from build123d import *

# Parameters (mm, degrees)
F1_DEPTH = 33
F2_R     = 1.1
F2_R_2   = 2
F3_DEPTH = 32.301
F4_R     = 1
F5_R     = 5


with BuildPart() as f1:
    # F0 (on Front) → F1 (new body)
    with BuildSketch(Plane.XZ):
        Polygon((0, 24.5), (0, 0), (1.5, 0), (1.5, 23), (30.8, 23), (30.8, 0), (32.3, 0), (32.3, 24.5), align=None)
    extrude(amount=F1_DEPTH)

    # F2 (on face) → F3 (cut, through all)
    with BuildSketch(Plane(origin=(0, 0, 0), x_dir=(0, -1, 0), z_dir=(-1, 0, 0))):
        with BuildLine():
            Line((0, 8), (0, 0))
            Line((0, 0), (24.5, 0))
            Line((24.5, 0), (24.5, 8))
            Line((24.5, 8), (12.5, 8))
            Line((12.5, 8), (12.5, 10))
            ThreePointArc((12.5, 10), (8.5, 14), (4.5, 10))
            Line((4.5, 10), (4.5, 8))
            Line((4.5, 8), (0, 8))
        make_face()
        with Locations((14.7225396744, 10)):
            Circle(F2_R)
        with Locations((12.9, 14.4)):
            Circle(F2_R)
        with Locations((8.5, 16.2225396744)):
            Circle(F2_R)
        with Locations((4.1, 14.4)):
            Circle(F2_R)
        with Locations((2.2774603256, 10)):
            Circle(F2_R)
        with Locations((28.5, 3)):
            Circle(F2_R_2)
    extrude(amount=-F3_DEPTH, mode=Mode.SUBTRACT)

    # F4
    f4_edges = [f1.edges().sort_by_distance(p)[0] for p in [
        (0.75, -4.5, 8),
        (31.55, -4.5, 8),
        (0.75, -12.5, 8),
        (31.55, -12.5, 8),
        (31.55, 0, 8),
        (0.75, 0, 8),
        (0.75, -24.5, 0),
        (31.55, -24.5, 0),
        (0.75, -33, 0),
        (31.55, -33, 0),
    ]]
    fillet(f4_edges, radius=F4_R)

    # F5
    f5_edges = [f1.edges().sort_by_distance(p)[0] for p in [
        (0.75, -24.5, 8),
        (31.55, -24.5, 8),
    ]]
    fillet(f5_edges, radius=F5_R)


solid = f1.part
The model under review builds one solid part; all positions refer to its coordinate system, in mm. A direction names the side the tool comes from. Round coordinates to 2 decimals unless told otherwise and drop trailing zeros. Order: outer loops, then holes, each group sorted by start corner. A loop starts at its lowest first (then second) coordinate and runs counter-clockwise, first axis right, second up. Notation, with made-up numbers: (35, -4) -> (60, -4) arc R18 ccw to (60, 19) -> close; hole circle Ø6 at (10, 19.25). An arc over 180 degrees is marked (long way). Write item = value, one per line. Start each with the question number.
Item 1: Clearance check with flat-ended pins moving along their axes: pin 1 Ø5 at (x, y) = (15, -16.5) entering from -Z; pin 2 Ø0.8 at (x, y) = (1, -17) entering from -Z; pin 3 Ø1.6 at (x, z) = (31.5, 2) entering from +Y; pin 4 Ø12 at (y, z) = (-11, 4) entering from +X. State where each tip first meets the part, or that it passes through.
Item 2: Consider section D-D on y = -29. Write out the cut boundary in (x, z), plus the area to 3 significant figures.
Item 3: For faces 1 (the face through (32, -17, 8)), 2 (the face through (0.76, -12.785, 8.301)), 3 (the face through (31.54, -4.69, 15.33)), list the 3-axis set-ups (+Z, -Z, +X, -X, +Y, -Y) from which the entire face can be reached by the end or side of a thin tool; tool diameter is ignored.
Item 4: Consider section B-B on z = 18.25. Write out the cut boundary in (x, y), plus the area to 3 significant figures.
Item 5: Consider section C-C on z = 2.5. Write out the cut boundary in (x, y).
Item 6: Consider section A-A on y = -8.5. Write out the cut boundary in (x, z).
Item 7: For line 1 along Z through (x, y) = (1.1, -28.5); line 2 along Z through (x, y) = (3.5, -14); line 3 along X through (y, z) = (-18, 8.5), list the stretches that pass through material, from the lowest coordinate up.
Item 8: Mouldability with a two-part tool opening along Z and no side actions: class faces 4 (the face through (31.56, -12.801, 8.285)), 5 (the face through (31.54, -8.357, 17.313)), 6 (the face through (1, -24.5, 2)) as released by +Z, released by -Z, zero draft, split by the parting line, or undercut.
Conclusion:
q1.pin_1 = 23
q1.pin_2 = 8
q1.pin_3 = -24.5
q1.pin_4 = 32.3
q2.outline = (0, 0) -> (1.5, 0) -> (1.5, 1.06) -> (0, 1.06) -> close; (0, 4.94) -> (1.5, 4.94) -> (1.5, 23) -> (30.8, 23) -> (30.8, 4.94) -> (32.3, 4.94) -> (32.3, 24.5) -> (0, 24.5) -> close; (30.8, 0) -> (32.3, 0) -> (32.3, 1.06) -> (30.8, 1.06) -> close
q2.area = 106 mm2
q3.face_1 = -Z, +X, -X, +Y
q3.face_2 = -Z, +X, -X
q3.face_3 = +X, -X
q4.outline = (0, -33) -> (1.5, -33) -> (1.5, 0) -> (0, 0) -> close; (30.8, -33) -> (32.3, -33) -> (32.3, 0) -> (30.8, 0) -> close
q4.area = 99.0 mm2
q5.outline = (0, -33) -> (1.5, -33) -> (1.5, -30.44) -> (0, -30.44) -> close; (0, -26.56) -> (1.5, -26.56) -> (1.5, -24.5) -> (0, -24.5) -> close; (30.8, -33) -> (32.3, -33) -> (32.3, -30.44) -> (30.8, -30.44) -> close; (30.8, -26.56) -> (32.3, -26.56) -> (32.3, -24.5) -> (30.8, -24.5) -> close
q6.outline = (0, 14) -> (1.5, 14) -> (1.5, 15.12) -> (0, 15.12) -> close; (0, 17.32) -> (1.5, 17.32) -> (1.5, 23) -> (30.8, 23) -> (30.8, 17.32) -> (32.3, 17.32) -> (32.3, 24.5) -> (0, 24.5) -> close; (30.8, 14) -> (32.3, 14) -> (32.3, 15.12) -> (30.8, 15.12) -> close
q7.line_1 = 0 to 1, 5 to 24.5
q7.line_2 = 23 to 24.5
q7.line_3 = 0 to 1.5, 30.8 to 32.3
q8.face_4 = released by -Z
q8.face_5 = undercut
q8.face_6 = zero draft
